The listing builds one solid part. Answer for the finished solid, in the listing's coordinates (mm). Face numbers are marked on the shaded views. A direction names the side the tool comes from. Coordinates: 2 decimals unless noted, no trailing zeros. Order: outer loops, then holes, each group sorted by start corner. A loop starts at its lowest first (then second) coordinate and runs counter-clockwise, first axis right, second up. Notation, with made-up numbers: (68.25, 7.25) -> (92.25, 7.25) arc R23 cw to (92.25, 26.25) -> close; hole circle Ø5 at (-9, 72). An arc over 180 degrees is marked (long way). Answer in a Markdown table with one row per item.
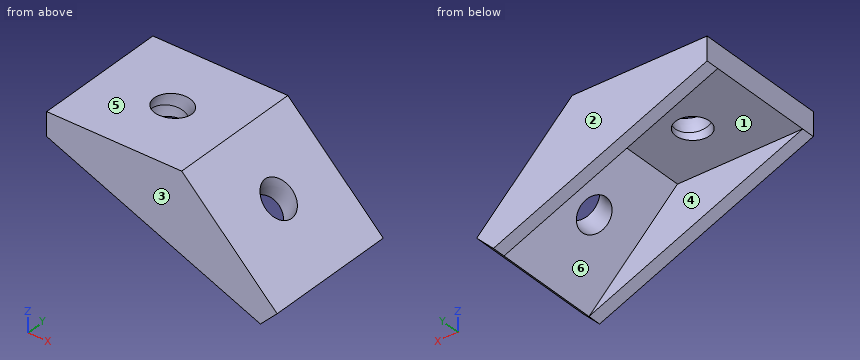
```python
from build123d import *

# Parameters (mm, degrees)
BOSS_EXTRUDE1_DEPTH = 20
BOSS_EXTRUDE2_DEPTH = 2
BOSS_EXTRUDE3_START = -20
BOSS_EXTRUDE3_DEPTH = 2
SKETCH3_R           = 2.5


with BuildPart() as part:
    # Sketch1 → Boss-Extrude1 (new body)
    with BuildSketch(Plane(origin=(0, 0, 0), x_dir=(1, 0, 0), z_dir=(0, 1, 0))):
        Polygon((-20, 3.5), (-1.449747468, 3.5), (11.66726189, 16.617009358), (14.142135624, 14.142135624), (0, 0), (-20, 0), align=None)
    extrude(amount=BOSS_EXTRUDE1_DEPTH)

    # Sketch2 → Boss-Extrude2 (add)
    with BuildSketch(Plane(origin=(0, 20, 0), x_dir=(1, 0, 0), z_dir=(0, 1, 0))):
        Polygon((-20, 3.5), (11.66726189, 16.617009358), (-1.449747468, 3.5), align=None)
    extrude(amount=-BOSS_EXTRUDE2_DEPTH)

    # Sketch2<2> → Boss-Extrude3 (add)
    with BuildSketch(Plane(origin=(0, 20, 0), x_dir=(1, 0, 0), z_dir=(0, 1, 0)).offset(BOSS_EXTRUDE3_START)):
        Polygon((-20, 3.5), (11.66726189, 16.617009358), (-1.449747468, 3.5), align=None)
    extrude(amount=BOSS_EXTRUDE3_DEPTH)

    # Sketch3 → Cut-Revolve1 (revolve, cut)
    with BuildSketch(Plane(origin=(0, 0, -3.5), x_dir=(-1, 0, 0), z_dir=(0, 0, -1)), mode=Mode.PRIVATE) as cut_revolve1_sk:
        with Locations((10, 10)):
            Circle(SKETCH3_R)
    revolve(cut_revolve1_sk.sketch.rotate(Axis((-1.449747468, 20, -3.5), (0, -1, 0)), 350.498874786), axis=Axis((-1.449747468, 20, -3.5), (0, -1, 0)), mode=Mode.SUBTRACT)


solid = part.part
```
(1) Flat-ended cylindrical pins translate along their axes: pin 1 (6 mm diameter, centred on x = 6.5, y = 7, fed in from -Z); pin 2 (5 mm diameter, centred on x = -13.5, y = 12, fed in from -Z); pin 3 (8 mm diameter, centred on x = 4, y = 8.5, fed in from -Z). Find the tip coordinate at first contact, or state that the pin passes through.
Check values:
| item | result |
|---|---|
| pin 1 | z = -14.45 |
| pin 2 | z = -3.5 |
| pin 3 | z = -12.95 |
(2) A cutting plane is placed at B-B, the plane x = 0.5. Determine the outline of the cut face in (y, z).
Check values:
| item | result |
|---|---|
| outline | (0, -11.99) -> (2, -11.99) -> (2, -5.45) -> (18, -5.45) -> (18, -11.99) -> (20, -11.99) -> (20, -0.5) -> (0, -0.5) -> close |
(3) Which of the six approach directions +Z, -Z, +X, -X, +Y, -Y give full straight-line access (tool end or side, diameter ignored) to the marked faces 1 and 2?
Check values:
| item | result |
|---|---|
| face 1 | -Z, -X |
| face 2 | +Z, -Z, +X, -X, +Y |
(4) For a pull along Y with two mould halves and no side action, classify the marked faces 3, 4, 5 and 6 as released by +Y, released by -Y, zero draft, split by the parting line, or undercut.
Check values:
| item | result |
|---|---|
| face 3 | released by -Y |
| face 4 | undercut |
| face 5 | zero draft |
| face 6 | undercut |
(5) A cutting plane is placed at A-A, the plane y = 8.75. Determine the outline of the cut face in (x, z).
Check values:
| item | result |
|---|---|
| outline | (-20, -3.5) -> (-12.17, -3.5) arc R10.72 cw to (-11.58, 0) -> (-20, 0) -> close; (-7.83, -3.5) -> (-1.45, -3.5) -> (3.07, -8.02) arc R6.39 ccw to (4.8, -4.8) -> (0, 0) -> (-6.79, 0) arc R6.39 ccw to start; (6.13, -11.08) -> (11.67, -16.62) -> (14.14, -14.14) -> (8.19, -8.19) arc R10.72 cw to start |
(6) Find the intervals of material crossed by line 1 along Y through (x, z) = (1, -10.25); line 2 along Z through (x, y) = (-14.5, 6); line 3 along Y through (x, z) = (6.5, -10), in increasing order. Write a range as from..to.
Check values:
| item | result |
|---|---|
| line 1 | 0..2, 18..20 |
| line 2 | -3.5..0 |
| line 3 | 0..8.18, 11.82..20 |
(7) A cutting plane is placed at D-D, the plane z = -15. Determine the outline of the cut face in (x, y), then the cut area to 3 significant figures.
Check values:
| item | result |
|---|---|
| outline | (7.76, 0) -> (13.28, 0) -> (13.28, 20) -> (7.76, 20) -> (7.76, 18) -> (10.05, 18) -> (10.05, 2) -> (7.76, 2) -> close |
| area | 73.8 mm² |
(8) A cutting plane is placed at C-C, the plane y = 15. Determine the outline of the cut face in (x, z).
Check values:
| item | result |
|---|---|
| outline | (-20, -3.5) -> (-1.45, -3.5) -> (11.67, -16.62) -> (14.14, -14.14) -> (0, 0) -> (-20, 0) -> close |
